Can you work these out from the drawing? Everything is in mm from the part's minimum corner. A direction names the side the tool comes from. Coordinates: 2 decimals unless noted, no trailing zeros. Order: outer loops, then holes, each group sorted by start corner. A loop starts at its lowest first (then second) coordinate and runs counter-clockwise, first axis right, second up. Notation, with made-up numbers: (7.25, 13.5) -> (20.25, 13.5) arc R33 ccw to (20.25, 49.5) -> close; hole circle Ø6 at (2.5, -18). An arc over 180 degrees is marked (long way). Use a Markdown table: item, result. Add a question column.
1) If we section it at D-D (z = 47.5): Write out the boundary of the cut face in (x, y).
2) If we section it at B-B (x = 10): Write out the boundary of the cut face in (y, z).
3) If we section it at A-A (z = 5): Write out the boundary of the cut face in (x, y), plus the area to 3 significant figures.
4) If I drill on L1, parallel to X at y = 8.25, z = 73; L2, parallel to X at y = 0.55, z = 69; L3, parallel to Y at x = 4, z = 22.5, over which ranges is the centre line in solid material (lowest first)? Write a range as [from, to].
5) Which directions (+Z, -Z, +X, -X, +Y, -Y) give clear straight access to the entire face, cutting with the end or side of a thin tool? Please do the marked faces 4 and 5.
6) Will this pin go through, and if not, where does the flat tip stop? pin 1 Ø3 at (x, z) = (10, 39) entering from +Y.
7) If we section it at C-C (y = 8): Write out the boundary of the cut face in (x, z), plus the area to 3 significant figures.
8) Thinking about a two-plate mould opening in X: for the marked faces 1, 2 and 3, which applies, +X half, -X half, draft (parallel to the pull), parting line (faces both ways), or undercut?
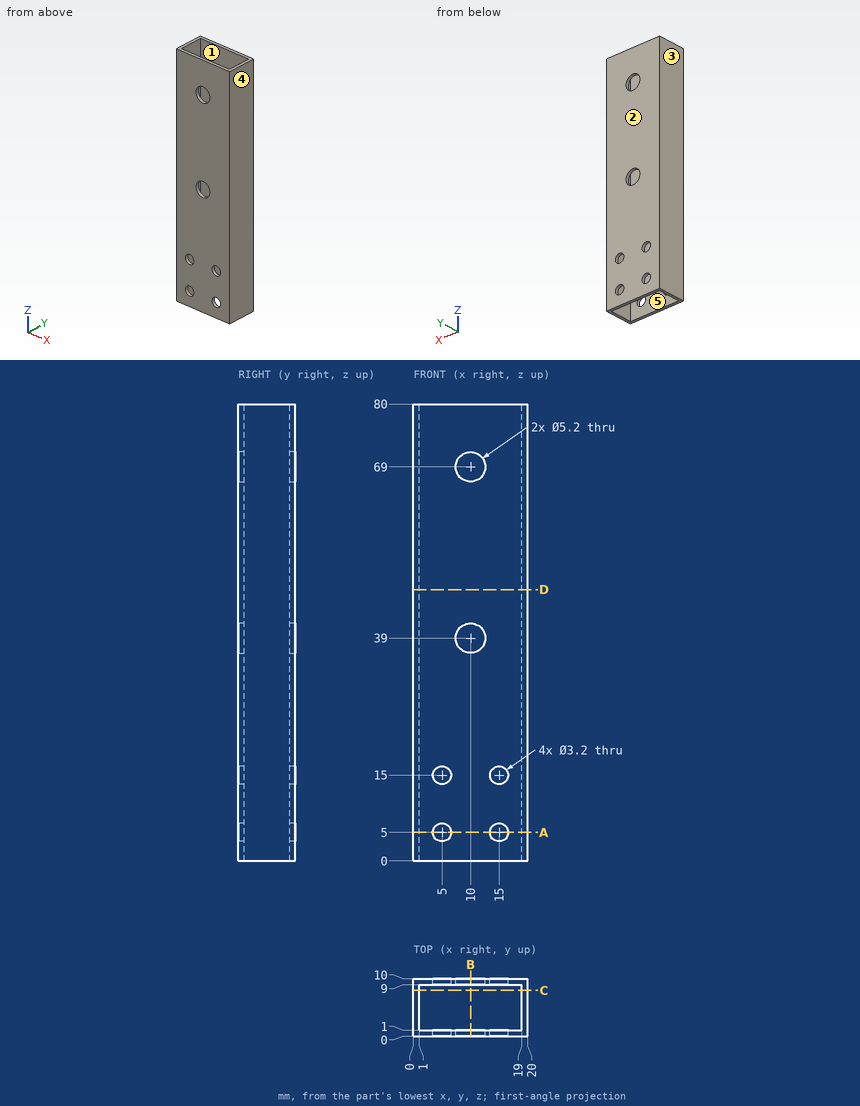
Answer sheet:
| question | item | result |
|---|---|---|
| 1 | outline | (0, 0) -> (20, 0) -> (20, 10) -> (0, 10) -> close; hole (1, 1) -> (19, 1) -> (19, 9) -> (1, 9) -> close |
| 2 | outline | (0, 0) -> (1, 0) -> (1, 36.4) -> (0, 36.4) -> close; (0, 41.6) -> (1, 41.6) -> (1, 66.4) -> (0, 66.4) -> close; (0, 71.6) -> (1, 71.6) -> (1, 80) -> (0, 80) -> close; (9, 0) -> (10, 0) -> (10, 36.4) -> (9, 36.4) -> close; (9, 41.6) -> (10, 41.6) -> (10, 66.4) -> (9, 66.4) -> close; (9, 71.6) -> (10, 71.6) -> (10, 80) -> (9, 80) -> close |
| 3 | outline | (0, 0) -> (3.4, 0) -> (3.4, 1) -> (1, 1) -> (1, 9) -> (3.4, 9) -> (3.4, 10) -> (0, 10) -> close; (6.6, 0) -> (13.4, 0) -> (13.4, 1) -> (6.6, 1) -> close; (6.6, 9) -> (13.4, 9) -> (13.4, 10) -> (6.6, 10) -> close; (16.6, 0) -> (20, 0) -> (20, 10) -> (16.6, 10) -> (16.6, 9) -> (19, 9) -> (19, 1) -> (16.6, 1) -> close |
| 3 | area | 43.2 mm2 |
| 4 | L1 | [0, 1], [19, 20] |
| 4 | L2 | [0, 7.4], [12.6, 20] |
| 4 | L3 | [0, 1], [9, 10] |
| 5 | face 4 | +Z, -Z, +X, +Y, -Y |
| 5 | face 5 | +Z, -Z |
| 6 | pin 1 | through |
| 7 | outline | (0, 0) -> (1, 0) -> (1, 80) -> (0, 80) -> close; (19, 0) -> (20, 0) -> (20, 80) -> (19, 80) -> close |
| 7 | area | 160 mm2 |
| 8 | face 1 | undercut |
| 8 | face 2 | draft |
| 8 | face 3 | -X half |
